Work out the finished part from the listing and answer in its coordinate system (mm). Face numbers are marked on the shaded views. A direction names the side the tool comes from. Give positions to 0.01 mm unless a question says otherwise; leave off trailing zeros. Order: outer loops, then holes, each group sorted by start corner. A loop starts at its lowest first (then second) coordinate and runs counter-clockwise, first axis right, second up. Notation, with made-up numbers: M 17,5 L 63,5 A35 cw 63,43 Z; hole C 20.25,-20 d6. An arc over 180 degrees is marked long. One line per item, written item: value.
from build123d import *
from build123d.topology import SkipClean

# Parameters (mm, degrees)
SKETCH_1_W           = 9.1
SKETCH_1_H           = 9.1
SKETCH_1_W_2         = 5.1
SKETCH_1_H_2         = 5.1
EXTRUDE_1_DEPTH      = 5
SKETCH_2_R           = 0.6
CUT_EXTRUDE_1_DEPTH  = 12.336335387
SKETCH_2_3_R         = 1
CUT_EXTRUDE_2_DEPTH  = 1
CUT_EXTRUDE_START    = -8.1
SKETCH_2_4_R         = 1
CUT_EXTRUDE_3_DEPTH  = 1
SKETCH_3_R           = 0.6
CUT_EXTRUDE_4_DEPTH  = 12.336335387
SKETCH_3_3_R         = 1
CUT_EXTRUDE_5_DEPTH  = 1
SKETCH_3_4_R         = 1
CUT_EXTRUDE_6_DEPTH  = 1
SKETCH_5_W           = 9.1
SKETCH_5_H           = 9.1
EXTRUDE_2_DEPTH      = 1
EXTRUDE_START        = 1
SKETCH_5_4_W         = 2.5
SKETCH_5_4_H         = 9.1
EXTRUDE_3_DEPTH      = 8
SKETCH_6_R           = 3
CUT_EXTRUDE_7_DEPTH  = 16.822215395
FILLET_1_R           = 3
CUT_EXTRUDE_11_REACH = 19.306
CUT_EXTRUDE_START_2  = -5.8
CUT_EXTRUDE_12_DEPTH = 3.3
EXTRUDE_4_DEPTH      = 3.3
EXTRUDE_START_2      = -5.8
EXTRUDE_5_DEPTH      = 3.3


with BuildPart() as part:
    # 草图1 → 凸台-拉伸1 (new body)
    with BuildSketch(Plane(origin=(0, 0, 0), x_dir=(1, 0, 0), z_dir=(0, 1, 0))):
        Rectangle(SKETCH_1_W, SKETCH_1_H)
        Rectangle(SKETCH_1_W_2, SKETCH_1_H_2, mode=Mode.SUBTRACT)
    extrude(amount=EXTRUDE_1_DEPTH)

    # 草图2 → 切除-拉伸1 (cut, through all)
    with BuildSketch(Plane.XY.offset(4.55)):
        with Locations((0, 2.5)):
            Circle(SKETCH_2_R)
    extrude(amount=-CUT_EXTRUDE_1_DEPTH, mode=Mode.SUBTRACT)

    # 草图2<3> → 切除-拉伸2 (cut)
    with BuildSketch(Plane.XY.offset(4.55)):
        with Locations((0, 2.5)):
            Circle(SKETCH_2_3_R)
    extrude(amount=-CUT_EXTRUDE_2_DEPTH, mode=Mode.SUBTRACT)

    # 草图2<4> → 切除-拉伸3 (cut)
    with BuildSketch(Plane.XY.offset(4.55).offset(CUT_EXTRUDE_START)):
        with Locations((0, 2.5)):
            Circle(SKETCH_2_4_R)
    extrude(amount=-CUT_EXTRUDE_3_DEPTH, mode=Mode.SUBTRACT)

    # 草图3 → 切除-拉伸4 (cut, through all)
    with BuildSketch(Plane.ZY.offset(4.55)):
        with Locations((0, 2.5)):
            Circle(SKETCH_3_R)
    extrude(amount=-CUT_EXTRUDE_4_DEPTH, mode=Mode.SUBTRACT)

    # 草图3<3> → 切除-拉伸5 (cut)
    with BuildSketch(Plane.ZY.offset(4.55)):
        with Locations((0, 2.5)):
            Circle(SKETCH_3_3_R)
    extrude(amount=-CUT_EXTRUDE_5_DEPTH, mode=Mode.SUBTRACT)

    # 草图3<4> → 切除-拉伸6 (cut)
    with BuildSketch(Plane.ZY.offset(4.55).offset(CUT_EXTRUDE_START)):
        with Locations((0, 2.5)):
            Circle(SKETCH_3_4_R)
    extrude(amount=-CUT_EXTRUDE_6_DEPTH, mode=Mode.SUBTRACT)

    # 草图5 → 凸台-拉伸2 (add)
    with BuildSketch(Plane(origin=(0, 5, 0), x_dir=(1, 0, 0), z_dir=(0, 1, 0))):
        Rectangle(SKETCH_5_W, SKETCH_5_H)
    extrude(amount=EXTRUDE_2_DEPTH)

    # 草图5<4> → 凸台-拉伸3 (add)
    with BuildSketch(Plane(origin=(0, 5, 0), x_dir=(1, 0, 0), z_dir=(0, 1, 0)).offset(EXTRUDE_START)):
        Rectangle(SKETCH_5_4_W, SKETCH_5_4_H)
    extrude(amount=EXTRUDE_3_DEPTH)

    # 草图6 → 切除-拉伸7 (cut, through all)
    with BuildSketch(Plane(origin=(1.25, 0, 0), x_dir=(0, 0, -1), z_dir=(1, 0, 0))):
        with Locations((0, 10)):
            Circle(SKETCH_6_R)
    extrude(amount=-CUT_EXTRUDE_7_DEPTH, mode=Mode.SUBTRACT)

    # 圆角1
    fillet_1_edges = [part.edges().sort_by_distance(p)[0] for p in [
        (0, 14, 4.55),
        (0, 14, -4.55),
    ]]
    fillet(fillet_1_edges, radius=FILLET_1_R)

    # 切除-拉伸11: up to this face of the body (flat: up to its plane)
    cut_extrude_11_end = Plane(part.part.faces().sort_by_distance((1.25, 8.5, 4.428834823))[0])
    # 草图7 → 切除-拉伸11 (cut, up to the picked face)
    with BuildSketch(Plane(origin=(4.55, 0, 0), x_dir=(0, 0, -1), z_dir=(1, 0, 0)), mode=Mode.PRIVATE) as cut_extrude_11_sk1:
        with BuildLine():
            ThreePointArc((5.5, 10), (-1.616322988, 15.257138005), (-4.55, 6.910097089))
            ThreePointArc((-4.55, 6.910097089), (-4.187258154, 6.43392805), (-3.774917218, 6))
            Line((-3.774917218, 6), (3.774917218, 6))
            ThreePointArc((3.774917218, 6), (4.187258154, 6.43392805), (4.55, 6.910097089))
            ThreePointArc((4.55, 6.910097089), (5.257138005, 8.383677012), (5.5, 10))
        make_face()
    cut_extrude_11_tool1 = split(extrude(cut_extrude_11_sk1.sketch, amount=-CUT_EXTRUDE_11_REACH, mode=Mode.PRIVATE), bisect_by=cut_extrude_11_end, keep=Keep.BOTH, mode=Mode.PRIVATE)
    # 草图7 → 切除-拉伸11 (cut, up to the picked face)
    with BuildSketch(Plane(origin=(4.55, 0, 0), x_dir=(0, 0, -1), z_dir=(1, 0, 0)), mode=Mode.PRIVATE) as cut_extrude_11_sk2:
        with BuildLine():
            Line((3.774917218, 6), (-3.774917218, 6))
            ThreePointArc((-3.774917218, 6), (0, 4.5), (3.774917218, 6))
        make_face()
    cut_extrude_11_tool2 = split(extrude(cut_extrude_11_sk2.sketch, amount=-CUT_EXTRUDE_11_REACH, mode=Mode.PRIVATE), bisect_by=cut_extrude_11_end, keep=Keep.BOTH, mode=Mode.PRIVATE)
    add(cut_extrude_11_tool1.solids().sort_by(Axis((4.55, 10.411022, 0), (-1, 0, 0)))[0], mode=Mode.SUBTRACT)
    add(cut_extrude_11_tool2.solids().sort_by(Axis((4.55, 5.392383, 0), (-1, 0, 0)))[0], mode=Mode.SUBTRACT)

    # 草图7<2> → 切除-拉伸12 (cut)
    with BuildSketch(Plane(origin=(4.55, 0, 0), x_dir=(0, 0, -1), z_dir=(1, 0, 0)).offset(CUT_EXTRUDE_START_2)):
        with BuildLine():
            ThreePointArc((5.5, 10), (-1.616322988, 15.257138005), (-4.55, 6.910097089))
            ThreePointArc((-4.55, 6.910097089), (-4.187258154, 6.43392805), (-3.774917218, 6))
            Line((-3.774917218, 6), (3.774917218, 6))
            ThreePointArc((3.774917218, 6), (4.187258154, 6.43392805), (4.55, 6.910097089))
            ThreePointArc((4.55, 6.910097089), (5.257138005, 8.383677012), (5.5, 10))
        make_face()
        with BuildLine():
            Line((3.774917218, 6), (-3.774917218, 6))
            ThreePointArc((-3.774917218, 6), (0, 4.5), (3.774917218, 6))
        make_face()
    extrude(amount=-CUT_EXTRUDE_12_DEPTH, mode=Mode.SUBTRACT)

    # 草图7<5> → 凸台-拉伸4 (add)
    with SkipClean():  # the faces are left unmerged after this step: merging them gives an invalid solid
        with BuildSketch(Plane(origin=(4.55, 0, 0), x_dir=(0, 0, -1), z_dir=(1, 0, 0))):
            with BuildLine():
                ThreePointArc((-3.774917218, 6), (-4.187258154, 6.43392805), (-4.55, 6.910097089))
                Line((-4.55, 6.910097089), (-4.55, 6))
                Line((-4.55, 6), (-3.774917218, 6))
            make_face()
            with BuildLine():
                Line((4.55, 6), (4.55, 6.910097089))
                ThreePointArc((4.55, 6.910097089), (4.187258154, 6.43392805), (3.774917218, 6))
                Line((3.774917218, 6), (4.55, 6))
            make_face()
        extrude(amount=-EXTRUDE_4_DEPTH)

    # 草图7<6> → 凸台-拉伸5 (add)
    with SkipClean():  # the faces are left unmerged after this step: merging them gives an invalid solid
        with BuildSketch(Plane(origin=(4.55, 0, 0), x_dir=(0, 0, -1), z_dir=(1, 0, 0)).offset(EXTRUDE_START_2)):
            with BuildLine():
                ThreePointArc((-3.774917218, 6), (-4.187258154, 6.43392805), (-4.55, 6.910097089))
                Line((-4.55, 6.910097089), (-4.55, 6))
                Line((-4.55, 6), (-3.774917218, 6))
            make_face()
            with BuildLine():
                Line((4.55, 6), (4.55, 6.910097089))
                ThreePointArc((4.55, 6.910097089), (4.187258154, 6.43392805), (3.774917218, 6))
                Line((3.774917218, 6), (4.55, 6))
            make_face()
        extrude(amount=-EXTRUDE_5_DEPTH)


solid = part.part
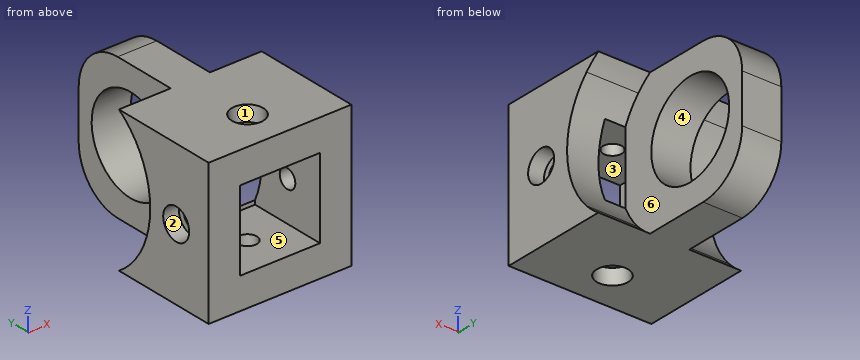
(1) Section A-A, the plane x = 0 is taken. Give the vertices of the cut face in (y, z), then the cut area to 3 significant figures.
Findings:
outline: M 0,-4.55 L 1.5,-4.55 L 1.5,-3.55 L 1.9,-3.55 L 1.9,-2.55 L 0,-2.55 Z; M 0,2.55 L 1.9,2.55 L 1.9,3.55 L 1.5,3.55 L 1.5,4.55 L 0,4.55 Z; M 3.1,-3.55 L 3.5,-3.55 L 3.5,-4.55 L 11,-4.55 A3 ccw 14,-1.55 L 14,1.55 A3 ccw 11,4.55 L 3.5,4.55 L 3.5,3.55 L 3.1,3.55 L 3.1,2.55 L 5,2.55 L 5,-2.55 L 3.1,-2.55 Z; hole C 10,0 d6
area: 63.4 mm^2
(2) Find the intervals of material crossed by probe 1 along X at (y, z) = (1.5, -2.5); probe 2 along Y at (x, z) = (-0.55, 0); probe 3 along Y at (x, z) = (-2.75, 0), in increasing order. Write a range as from..to.
Findings:
probe 1: x = -4.55..-2.55, 2.55..4.55
probe 2: y = 5..7, 13..14
probe 3: y = 0..1.9, 3.1..4.5
(3) Given P1, Ø0.6, axis at y = 2.5, z = -0.5, coming from the +X side; P2, Ø1.5, axis at y = 6.5, z = 0.5, coming from the +X side; P3, Ø1, axis at x = 0, y = 2.5, coming from the -Z side; P4, Ø1.6, axis at x = 0, y = 2.5, coming from the +Z side, each flat-ended and moving along its own axis, determine where each tip first touches the part or whether it passes through.
Findings:
P1: stops at x = 3.55
P2: stops at x = 1.25
P3: passes through
P4: stops at z = 3.55
(4) Section B-B, the plane z = 0 is taken. Give the number of separate pieces and of enclosed holes in the cut face, then the cut area to 3 significant figures.
Findings:
separate pieces: 6
enclosed holes: 0
area: 19.1 mm^2
(5) Determine the mould class of the marked faces 4, 5 and 6 for opening direction X: pulls with the +X half, pulls with the -X half, needs draft (parallel to the pull), parting line crosses it, or undercut.
Findings:
face 4: needs draft
face 5: undercut
face 6: pulls with the +X half
(6) Section C-C, the plane x = 3.25 is taken. Give the vertices of the cut face in (y, z), then the cut area to 3 significant figures.
Findings:
outline: M 0,-4.55 L 6.91,-4.55 A5.5 cw 6.91,4.55 L 0,4.55 Z; hole C 2.5,0 d1.2
area: 46.3 mm^2
(7) Which of the six approach directions +Z, -Z, +X, -X, +Y, -Y give full straight-line access (tool end or side, diameter ignored) to the marked faces 1, 2 and 3?
Findings:
face 1: +Z
face 2: -X
face 3: -Y
